Check sheet for the modelled part. Datum: model origin and axes. Units: mm. Give positions to 0.01 mm unless a question says otherwise; leave off trailing zeros. Loops run counter-clockwise (first coordinate to the right, second up) from the corner with the lowest first, then second, coordinate; pieces in that order, holes last. Notation, with made-up numbers: (12.5, 63.5) - (29.5, 63.5) arc R33 cw to (29.5, 97.5) - close; hole circle Ø9 at (31, 49.5). An arc over 180 degrees is marked (long way). Answer in a Markdown table with one row per item. Add a question column.
(1) Sectioned sample at C-C on z = 2.1. State how many separate pieces and enclosed holes the cut face has, then the cut area to 3 significant figures.
(2) Sectioned sample at A-A on x = 3.5. Enter the section's corners in (y, z), then the cut area to 3 significant figures.
(3) Thickness scan on L1, parallel to X at y = 27.5, z = 3.4; L2, parallel to Y at x = -62, z = 2.2; L3, parallel to X at y = -39, z = 0.75. Record the ranges inside material, lowest first.
(4) Sectioned sample at D-D on y = 62. Enter the section's corners in (x, z), then the cut area to 3 significant figures.
(5) Go/stop test with flat-tipped pins: P1, Ø4, axis at x = -23.5, y = 25.5, coming from the -Z side; P2, Ø2.5, axis at x = -25, y = 25, coming from the +Z side. Record where each tip stops, or that it passes through.
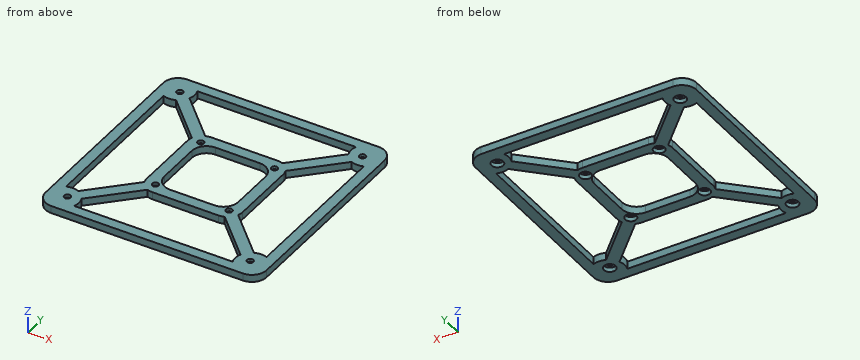
from build123d import *

# Parameters (mm, degrees)
SKETCH1_R             = 11
BOSS_EXTRUDE1_DEPTH   = 5
BOSS_EXTRUDE1_2_DEPTH = 5
BOSS_EXTRUDE1_3_DEPTH = 5
BOSS_EXTRUDE1_4_DEPTH = 5
SKETCH3_W             = 150
SKETCH3_H             = 150
SKETCH3_W_2           = 136
SKETCH3_H_2           = 136
BOSS_EXTRUDE3_DEPTH   = 5
SKETCH8_R             = 2.14
BOSS_EXTRUDE4_DEPTH   = 5
BOSS_EXTRUDE4_2_DEPTH = 5
BOSS_EXTRUDE4_3_DEPTH = 5
BOSS_EXTRUDE4_4_DEPTH = 5
FILLET1_R             = 10
SKETCH9_R             = 4
BOSS_EXTRUDE5_DEPTH   = 3
BOSS_EXTRUDE5_2_DEPTH = 3
BOSS_EXTRUDE5_3_DEPTH = 3
BOSS_EXTRUDE5_4_DEPTH = 3
SKETCH10_W            = 65
SKETCH10_H            = 65
SKETCH10_W_2          = 50
SKETCH10_H_2          = 50
BOSS_EXTRUDE6_DEPTH   = 5
FILLET2_R             = 10
SKETCH11_R            = 2.14
BOSS_EXTRUDE7_DEPTH   = 5
BOSS_EXTRUDE7_2_DEPTH = 5
BOSS_EXTRUDE7_3_DEPTH = 5
BOSS_EXTRUDE7_4_DEPTH = 5
SKETCH12_R            = 3.8
BOSS_EXTRUDE8_DEPTH   = 3
BOSS_EXTRUDE8_2_DEPTH = 3
BOSS_EXTRUDE8_3_DEPTH = 3
BOSS_EXTRUDE8_4_DEPTH = 3
BOSS_EXTRUDE9_DEPTH   = 5
BOSS_EXTRUDE9_2_DEPTH = 5
BOSS_EXTRUDE9_3_DEPTH = 5
BOSS_EXTRUDE9_4_DEPTH = 5


with BuildPart() as part:
    # Sketch1 → Boss-Extrude1 (new body)
    with BuildSketch(Plane.XY):
        with Locations((-64, -64)):
            Circle(SKETCH1_R)
    extrude(amount=BOSS_EXTRUDE1_DEPTH)


with BuildPart() as body_2:
    # Sketch1 → Boss-Extrude1 2 (new body)
    with BuildSketch(Plane.XY):
        with Locations((-64, 64)):
            Circle(SKETCH1_R)
    extrude(amount=BOSS_EXTRUDE1_2_DEPTH)



with BuildPart() as body_3:
    # Sketch1 → Boss-Extrude1 3 (new body)
    with BuildSketch(Plane.XY):
        with Locations((64, -64)):
            Circle(SKETCH1_R)
    extrude(amount=BOSS_EXTRUDE1_3_DEPTH)


with BuildPart() as body_4:
    # Sketch1 → Boss-Extrude1 4 (new body)
    with BuildSketch(Plane.XY):
        with Locations((64, 64)):
            Circle(SKETCH1_R)
    extrude(amount=BOSS_EXTRUDE1_4_DEPTH)


with BuildPart() as body_2_1:
    add(body_2.part)

    add(body_3.part)  # Boss-Extrude3 merges body 3

    add(body_4.part)  # Boss-Extrude3 merges body 4
    # Sketch3 → Boss-Extrude3 (add)
    with BuildSketch(Plane.XY):
        Rectangle(SKETCH3_W, SKETCH3_H)
        Rectangle(SKETCH3_W_2, SKETCH3_H_2, mode=Mode.SUBTRACT)
    extrude(amount=BOSS_EXTRUDE3_DEPTH)

    # Fillet1
    fillet1_edges = [body_2_1.edges().sort_by_distance(p)[0] for p in [
        (75, -75, 2.5),
        (75, 75, 2.5),
        (-75, 75, 2.5),
        (-75, -75, 2.5),
    ]]
    fillet(fillet1_edges, radius=FILLET1_R)

    # Combine1: union part
    add(part.part)


with BuildPart() as body_3_2:
    # Sketch8 → Boss-Extrude4 (new body)
    with BuildSketch(Plane.XY):
        with Locations((-62, 62)):
            Circle(SKETCH8_R)
    extrude(amount=BOSS_EXTRUDE4_DEPTH)


with BuildPart() as body_4_2:
    # Sketch8 → Boss-Extrude4 2 (new body)
    with BuildSketch(Plane.XY):
        with Locations((-62, -62)):
            Circle(SKETCH8_R)
    extrude(amount=BOSS_EXTRUDE4_2_DEPTH)


with BuildPart() as body_5:
    # Sketch8 → Boss-Extrude4 3 (new body)
    with BuildSketch(Plane.XY):
        with Locations((62, 62)):
            Circle(SKETCH8_R)
    extrude(amount=BOSS_EXTRUDE4_3_DEPTH)


with BuildPart() as body_6:
    # Sketch8 → Boss-Extrude4 4 (new body)
    with BuildSketch(Plane.XY):
        with Locations((62, -62)):
            Circle(SKETCH8_R)
    extrude(amount=BOSS_EXTRUDE4_4_DEPTH)


with BuildPart() as body_6_2:
    # Sketch9 → Boss-Extrude5 (new body)
    with BuildSketch(Plane.XY):
        with Locations((-62, 62)):
            Circle(SKETCH9_R)
    extrude(amount=BOSS_EXTRUDE5_DEPTH)


with BuildPart() as body_7:
    # Sketch9 → Boss-Extrude5 2 (new body)
    with BuildSketch(Plane.XY):
        with Locations((-62, -62)):
            Circle(SKETCH9_R)
    extrude(amount=BOSS_EXTRUDE5_2_DEPTH)


with BuildPart() as body_8:
    # Sketch9 → Boss-Extrude5 3 (new body)
    with BuildSketch(Plane.XY):
        with Locations((62, 62)):
            Circle(SKETCH9_R)
    extrude(amount=BOSS_EXTRUDE5_3_DEPTH)


with BuildPart() as body_9:
    # Sketch9 → Boss-Extrude5 4 (new body)
    with BuildSketch(Plane.XY):
        with Locations((62, -62)):
            Circle(SKETCH9_R)
    extrude(amount=BOSS_EXTRUDE5_4_DEPTH)


with BuildPart() as body_10:
    # Sketch10 → Boss-Extrude6 (new body)
    with BuildSketch(Plane.XY):
        Rectangle(SKETCH10_W, SKETCH10_H)
        Rectangle(SKETCH10_W_2, SKETCH10_H_2, mode=Mode.SUBTRACT)
    extrude(amount=BOSS_EXTRUDE6_DEPTH)

    # Fillet2
    fillet2_edges = [body_10.edges().sort_by_distance(p)[0] for p in [
        (-25, -25, 2.5),
        (25, -25, 2.5),
        (-25, 25, 2.5),
        (25, 25, 2.5),
        (32.5, -32.5, 2.5),
        (-32.5, -32.5, 2.5),
        (-32.5, 32.5, 2.5),
        (32.5, 32.5, 2.5),
    ]]
    fillet(fillet2_edges, radius=FILLET2_R)


with BuildPart() as body_11:
    # Sketch11 → Boss-Extrude7 (new body)
    with BuildSketch(Plane.XY):
        with Locations((25, 25)):
            Circle(SKETCH11_R)
    extrude(amount=BOSS_EXTRUDE7_DEPTH)


with BuildPart() as body_12:
    # Sketch11 → Boss-Extrude7 2 (new body)
    with BuildSketch(Plane.XY):
        with Locations((-25, 25)):
            Circle(SKETCH11_R)
    extrude(amount=BOSS_EXTRUDE7_2_DEPTH)


with BuildPart() as body_13:
    # Sketch11 → Boss-Extrude7 3 (new body)
    with BuildSketch(Plane.XY):
        with Locations((-25, -25)):
            Circle(SKETCH11_R)
    extrude(amount=BOSS_EXTRUDE7_3_DEPTH)


with BuildPart() as body_14:
    # Sketch11 → Boss-Extrude7 4 (new body)
    with BuildSketch(Plane.XY):
        with Locations((25, -25)):
            Circle(SKETCH11_R)
    extrude(amount=BOSS_EXTRUDE7_4_DEPTH)


with BuildPart() as body_15:
    # Sketch12 → Boss-Extrude8 (new body)
    with BuildSketch(Plane.XY):
        with Locations((25, 25)):
            Circle(SKETCH12_R)
    extrude(amount=BOSS_EXTRUDE8_DEPTH)


with BuildPart() as body_16:
    # Sketch12 → Boss-Extrude8 2 (new body)
    with BuildSketch(Plane.XY):
        with Locations((-25, 25)):
            Circle(SKETCH12_R)
    extrude(amount=BOSS_EXTRUDE8_2_DEPTH)


with BuildPart() as body_17:
    # Sketch12 → Boss-Extrude8 3 (new body)
    with BuildSketch(Plane.XY):
        with Locations((-25, -25)):
            Circle(SKETCH12_R)
    extrude(amount=BOSS_EXTRUDE8_3_DEPTH)


with BuildPart() as body_18:
    # Sketch12 → Boss-Extrude8 4 (new body)
    with BuildSketch(Plane.XY):
        with Locations((25, -25)):
            Circle(SKETCH12_R)
    extrude(amount=BOSS_EXTRUDE8_4_DEPTH)


with BuildPart() as body_19:
    # Sketch14 → Boss-Extrude9 (new body)
    with BuildSketch(Plane.XY):
        with BuildLine():
            Line((-59.171572875, 64.828427125), (-22.171572875, 27.828427125))
            ThreePointArc((-22.171572875, 27.828427125), (-22.171572875, 22.171572875), (-27.828427125, 22.171572875))
            Line((-27.828427125, 22.171572875), (-64.828427125, 59.171572875))
            ThreePointArc((-64.828427125, 59.171572875), (-64.828427125, 64.828427125), (-59.171572875, 64.828427125))
        make_face()
    extrude(amount=BOSS_EXTRUDE9_DEPTH)


with BuildPart() as body_20:
    # Sketch14 → Boss-Extrude9 2 (new body)
    with BuildSketch(Plane.XY):
        with BuildLine():
            Line((64.828427125, 59.171572875), (27.828427125, 22.171572875))
            ThreePointArc((27.828427125, 22.171572875), (22.171572875, 22.171572875), (22.171572875, 27.828427125))
            Line((22.171572875, 27.828427125), (59.171572875, 64.828427125))
            ThreePointArc((59.171572875, 64.828427125), (64.828427125, 64.828427125), (64.828427125, 59.171572875))
        make_face()
    extrude(amount=BOSS_EXTRUDE9_2_DEPTH)


with BuildPart() as body_21:
    # Sketch14 → Boss-Extrude9 3 (new body)
    with BuildSketch(Plane.XY):
        with BuildLine():
            Line((27.828427125, -22.171572875), (64.828427125, -59.171572875))
            ThreePointArc((64.828427125, -59.171572875), (64.828427125, -64.828427125), (59.171572875, -64.828427125))
            Line((59.171572875, -64.828427125), (22.171572875, -27.828427125))
            ThreePointArc((22.171572875, -27.828427125), (22.171572875, -22.171572875), (27.828427125, -22.171572875))
        make_face()
    extrude(amount=BOSS_EXTRUDE9_3_DEPTH)


with BuildPart() as body_22:
    # Sketch14 → Boss-Extrude9 4 (new body)
    with BuildSketch(Plane.XY):
        with BuildLine():
            Line((-22.171572875, -27.828427125), (-59.171572875, -64.828427125))
            ThreePointArc((-59.171572875, -64.828427125), (-64.828427125, -64.828427125), (-64.828427125, -59.171572875))
            Line((-64.828427125, -59.171572875), (-27.828427125, -22.171572875))
            ThreePointArc((-27.828427125, -22.171572875), (-22.171572875, -22.171572875), (-22.171572875, -27.828427125))
        make_face()
    extrude(amount=BOSS_EXTRUDE9_4_DEPTH)

    # Combine4: union body 21, body 20, body 19, body 2, body 10
    add(body_21.part)
    add(body_20.part)
    add(body_19.part)
    add(body_2_1.part)
    add(body_10.part)

    # Combine5: cut body 15, body 18, body 17, body 16, body 11, body 14, body 13, body 12, body 9, body 6 2, body 8, body 7, body 6, body 3 2, body 5, body 4 2
    add(body_15.part, mode=Mode.SUBTRACT)
    add(body_18.part, mode=Mode.SUBTRACT)
    add(body_17.part, mode=Mode.SUBTRACT)
    add(body_16.part, mode=Mode.SUBTRACT)
    add(body_11.part, mode=Mode.SUBTRACT)
    add(body_14.part, mode=Mode.SUBTRACT)
    add(body_13.part, mode=Mode.SUBTRACT)
    add(body_12.part, mode=Mode.SUBTRACT)
    add(body_9.part, mode=Mode.SUBTRACT)
    add(body_6_2.part, mode=Mode.SUBTRACT)
    add(body_8.part, mode=Mode.SUBTRACT)
    add(body_7.part, mode=Mode.SUBTRACT)
    add(body_6.part, mode=Mode.SUBTRACT)
    add(body_3_2.part, mode=Mode.SUBTRACT)
    add(body_5.part, mode=Mode.SUBTRACT)
    add(body_4_2.part, mode=Mode.SUBTRACT)


solid = body_22.part
Reply:
| question | item | result |
|---|---|---|
| 1 | separate pieces | 1 |
| 1 | enclosed holes | 13 |
| 1 | area | 7,270 mm^2 |
| 2 | outline | (-75, 0) - (-68, 0) - (-68, 5) - (-75, 5) - close; (-32.5, 0) - (-25, 0) - (-25, 5) - (-32.5, 5) - close; (25, 0) - (32.5, 0) - (32.5, 5) - (25, 5) - close; (68, 0) - (75, 0) - (75, 5) - (68, 5) - close |
| 2 | area | 145 mm^2 |
| 3 | L1 | -75 to -68, -33.16 to 33.16, 68 to 75 |
| 3 | L2 | -75 to -66, -58 to -53.18, 53.18 to 58, 66 to 75 |
| 3 | L3 | -75 to -68, -44.66 to -33.34, 33.34 to 44.66, 68 to 75 |
| 4 | outline | (-75, 0) - (-66, 0) - (-66, 3) - (-64.14, 3) - (-64.14, 5) - (-75, 5) - close; (-59.86, 3) - (-58, 3) - (-58, 0) - (-53.18, 0) - (-53.18, 5) - (-59.86, 5) - close; (53.18, 0) - (58, 0) - (58, 3) - (59.86, 3) - (59.86, 5) - (53.18, 5) - close; (64.14, 3) - (66, 3) - (66, 0) - (75, 0) - (75, 5) - (64.14, 5) - close |
| 4 | area | 153 mm^2 |
| 5 | P1 | z = 3 |
| 5 | P2 | through |
